from build123d import *

# Parameters (mm, degrees)
BOSS_EXTRUDE1_DEPTH = 20
CUT_EXTRUDE1_DEPTH  = 15
FILLET1_R           = 2
SKETCH5_R           = 1.5
CUT_EXTRUDE4_DEPTH  = 32.535079673
SCALE1_SCALE        = 1.02


with BuildPart() as part:
    # Sketch1 → Boss-Extrude1 (new body)
    with BuildSketch(Plane(origin=(0, 0, 0), x_dir=(0, 0, -1), z_dir=(1, 0, 0))):
        Polygon((0, -12.5), (-3.175, -12.5), (-6.175, -12.5), (-6.175, 15.675), (-3.175, 15.675), (0, 15.675), (3, 15.675), (12.5, 6.175), (12.5, 3.175), (12.5, 0), (12.5, -3), (3, -12.5), align=None)
    extrude(amount=BOSS_EXTRUDE1_DEPTH)

    # Sketch2 → Cut-Extrude1 (cut)
    with BuildSketch(Plane(origin=(20, 0, 0), x_dir=(0, 0, -1), z_dir=(1, 0, 0))):
        Polygon((-3.175, -12.5), (0, -12.5), (0, 0), (12.5, 0), (12.5, 3.175), (0, 3.175), (0, 15.675), (-3.175, 15.675), (-3.175, 3.175), align=None)
    extrude(amount=-CUT_EXTRUDE1_DEPTH, mode=Mode.SUBTRACT)

    # Fillet1
    fillet1_edges = [part.edges().sort_by_distance(p)[0] for p in [
        (20, 1.5875, 3.175),
        (20, -6.25, 0),
        (20, 0, -6.25),
        (20, 3.175, -6.25),
        (20, 9.425, 0),
    ]]
    fillet(fillet1_edges, radius=FILLET1_R)

    # Sketch5 → Cut-Extrude4 (cut, through all)
    with BuildSketch(Plane.XY.offset(6.175)):
        with Locations(Location((12.5, 9.175, 0), (0, 0, 90))):
            Circle(SKETCH5_R)
        with Locations(Location((12.5, -6, 0), (0, 0, 90))):
            Circle(SKETCH5_R)
    extrude(amount=-CUT_EXTRUDE4_DEPTH, mode=Mode.SUBTRACT)


with BuildPart() as part_1:
    # Scale1: scaled about (9.096060395, 1.5875, -2.193637699)
    add(part.part.scale(SCALE1_SCALE).moved(Location((-0.181921208, -0.03175, 0.043872754))))


solid = part_1.part
Geometry: final body of the model. Coordinates: model frame, mm. A direction names the side the tool comes from. Give positions to 0.01 mm unless a question says otherwise; leave off trailing zeros. Write each loop counter-clockwise with the first axis right and the second up, starting at its lowest first coordinate (ties: lowest second). Pieces come first, ordered by that corner, then holes. Notation, with made-up numbers: M 79.25,23.5 L 105.25,23.5 A29 cw 105.25,47.5 Z; hole C 30,79.25 d5. An arc over 180 degrees is marked long. Answer in a Markdown table with one row per item. Add a question column.
(1) Reachability of faces 4 (the flat face through (10, 4, -12.706)), 5 (the cylindrical face through (19.605, 9.671, -0.538)), 6 (the flat face through (12, -0.032, -6)) from +Z, -Z, +X, -X, +Y, -Y: full face, straight path, thin tool, end or side. Return the list, or none.
(2) Section B-B on z = -6.75. Return loops of the section in (x, y), and give its area (3 significant figures).
(3) Ray query, line 1 (Y direction, x = 12.5, z = -6.75); line 2 (Y direction, x = 6.5, z = 0); line 3 (Z direction, x = 8, y = 0.5). Return the intervals inside material, ascending.
(4) Section C-C on x = 13. State how many separate pieces and enclosed holes the cut face has, and give its area (3 significant figures).
(5) First-contact query: pin 1 (1.8 mm diameter, centred on x = 12.57, y = -6.15, fed in from +Z); pin 2 (5 mm diameter, centred on x = 12.57, y = -6.15, fed in from -Z); pin 3 (2 mm diameter, centred on x = 12, z = -8, fed in from +Y); pin 4 (1 mm diameter, centred on x = 3, y = -7, fed in from -Z). Flat tips, straight axial feed; report the tip coordinate or a pass-through.
(6) Section D-D on y = -0.75. Return loops of the section in (x, z), and give its area (3 significant figures).
(7) Mould query, pull axis Y, two halves, no side actions, for faces 1 (the flat face through (20.218, 2, 6)), 2 (the cylindrical face through (13.154, -4.738, -4.241)), 3 (the flat face through (9.9, -7.9, -7.9)). Classes: +Y half, -Y half, draft (parallel to the pull), parting line (faces both ways), or undercut.
(8) Section A-A on x = 6. Return loops of the section in (y, z), and give its area (3 significant figures).
Result set:
| question | item | result |
|---|---|---|
| 1 | face 4 | -Z, +X, -X, +Y, -Y |
| 1 | face 5 | +X, +Y, -Y |
| 1 | face 6 | -Z, +X |
| 2 | outline | M -0.18,-9.05 L 20.22,-9.05 L 20.22,-2.07 A2.04 ccw 18.18,-0.03 L 4.92,-0.03 L 4.92,3.21 L 18.18,3.21 A2.04 ccw 20.22,5.25 L 20.22,12.22 L -0.18,12.22 Z; hole C 12.57,-6.15 d3.06; hole C 12.57,9.33 d3.06 |
| 2 | area | 368 mm^2 |
| 3 | line 1 | y = -9.05 to -7.68, -4.62 to -0.03, 3.21 to 7.8, 10.86 to 12.22 |
| 3 | line 2 | y = -12.78 to -0.03, 3.21 to 15.96 |
| 3 | line 3 | z = 3.28 to 6.34 |
| 4 | separate pieces | 7 |
| 4 | enclosed holes | 0 |
| 4 | area | 244 mm^2 |
| 5 | pin 1 | passes through |
| 5 | pin 2 | stops at z = -12.15 |
| 5 | pin 3 | stops at y = 11.97 |
| 5 | pin 4 | stops at z = -9.3 |
| 6 | outline | M -0.18,-12.71 L 19.73,-12.71 L 19.73,-0.67 A2.04 ccw 18.18,0.04 L 4.92,0.04 L 4.92,3.28 L 18.18,3.28 A2.04 ccw 20.22,5.32 L 20.22,6.34 L -0.18,6.34 Z |
| 6 | area | 332 mm^2 |
| 7 | face 1 | draft |
| 7 | face 2 | undercut |
| 7 | face 3 | -Y half |
| 8 | outline | M -12.78,-3.02 L -3.09,-12.71 L -0.03,-12.71 L -0.03,0.04 L -12.78,0.04 Z; M -12.78,3.28 L 15.96,3.28 L 15.96,6.34 L -12.78,6.34 Z; M 3.21,-12.71 L 6.27,-12.71 L 15.96,-3.02 L 15.96,0.04 L 3.21,0.04 Z |
| 8 | area | 319 mm^2 |
